```python
from build123d import *

# Parameters (mm, degrees)
SALIENTE_EXTRUIR1_DEPTH = 37
SALIENTE_EXTRUIR2_DEPTH = 2
CROQUIS3_R              = 6.5
SALIENTE_EXTRUIR3_DEPTH = 1
CROQUIS4_R              = 5.5
SALIENTE_EXTRUIR4_DEPTH = 0.5
CROQUIS5_R              = 2.75
SALIENTE_EXTRUIR5_DEPTH = 4
CROQUIS7_W              = 11.5
CROQUIS7_H              = 16.4
SALIENTE_EXTRUIR6_DEPTH = 0.3
REDONDEO1_R             = 0.1
REDONDEO2_R             = 0.5
SALIENTE_EXTRUIR7_START = -8.45
SALIENTE_EXTRUIR7_DEPTH = 2.45
SALIENTE_EXTRUIR8_DEPTH = 0.5
CROQUIS11_W             = 6
CROQUIS11_H             = 2.5
SALIENTE_EXTRUIR9_DEPTH = 5
SALIENTE_EXTRUIR9_DRAFT = -8
CROQUIS12_R             = 1.25
CORTAR_EXTRUIR1_DEPTH   = 5
CHAFL_N1_SIZE           = 0.5


with BuildPart() as part:
    # Croquis1 → Saliente-Extruir1 (new body)
    with BuildSketch(Plane(origin=(0, 0, 0), x_dir=(1, 0, 0), z_dir=(0, 1, 0))):
        with BuildLine():
            Line((1, 0), (39, 0))
            ThreePointArc((39, 0), (39.707106781, 0.292893219), (40, 1))
            Line((40, 1), (40, 18))
            ThreePointArc((40, 18), (39.707106781, 18.707106781), (39, 19))
            Line((39, 19), (1, 19))
            ThreePointArc((1, 19), (0.292893219, 18.707106781), (0, 18))
            Line((0, 18), (0, 1))
            ThreePointArc((0, 1), (0.292893219, 0.292893219), (1, 0))
        make_face()
    extrude(amount=SALIENTE_EXTRUIR1_DEPTH)

    # Croquis2 → Saliente-Extruir2 (add)
    with BuildSketch(Plane(origin=(0, 37, 0), x_dir=(1, 0, 0), z_dir=(0, 1, 0))):
        with BuildLine():
            Line((13.315756806, 18.2), (34.5, 18.2))
            Line((34.5, 18.2), (34.5, 14.5))
            ThreePointArc((34.5, 14.5), (37.18337521, 9.5), (34.5, 4.5))
            Line((34.5, 4.5), (34.5, 0.8))
            Line((34.5, 0.8), (13.315756806, 0.8))
            ThreePointArc((13.315756806, 0.8), (0, 9.5), (13.315756806, 18.2))
        make_face()
    extrude(amount=SALIENTE_EXTRUIR2_DEPTH)

    # Croquis3 → Saliente-Extruir3 (add)
    with BuildSketch(Plane(origin=(0, 39, 0), x_dir=(1, 0, 0), z_dir=(0, 1, 0))):
        with Locations(Location((9.5, 9.5, 0), (0, 0, 270))):
            Circle(CROQUIS3_R)
    extrude(amount=SALIENTE_EXTRUIR3_DEPTH)

    # Croquis4 → Saliente-Extruir4 (add)
    with BuildSketch(Plane(origin=(0, 40, 0), x_dir=(1, 0, 0), z_dir=(0, 1, 0))):
        with Locations(Location((9.5, 9.5, 0), (0, 0, 270))):
            Circle(CROQUIS4_R)
    extrude(amount=SALIENTE_EXTRUIR4_DEPTH)

    # Croquis5 → Saliente-Extruir5 (add)
    with BuildSketch(Plane(origin=(0, 40.5, 0), x_dir=(1, 0, 0), z_dir=(0, 1, 0))):
        with Locations(Location((9.5, 9.5, 0), (0, 0, 270))):
            Circle(CROQUIS5_R)
    extrude(amount=SALIENTE_EXTRUIR5_DEPTH)

    # Croquis7 → Saliente-Extruir6 (add)
    with BuildSketch(Plane(origin=(0, 39, 0), x_dir=(1, 0, 0), z_dir=(0, 1, 0))):
        with BuildLine():
            Line((34.5, 0.8), (22, 0.8))
            Line((22, 0.8), (22, 8))
            ThreePointArc((22, 8), (20.5, 9.5), (22, 11))
            Line((22, 11), (22, 18.2))
            Line((22, 18.2), (34.5, 18.2))
            Line((34.5, 18.2), (34.5, 0.8))
        make_face()
        with Locations((28.25, 9.5)):
            Rectangle(CROQUIS7_W, CROQUIS7_H, mode=Mode.SUBTRACT)
    extrude(amount=SALIENTE_EXTRUIR6_DEPTH)

    # Redondeo1
    redondeo1_edges = [part.edges().sort_by_distance(p)[0] for p in [
        (34, 39.15, -1.3),
        (34, 39.15, -17.7),
        (22.5, 39.15, -17.7),
        (22.5, 39.15, -1.3),
    ]]
    fillet(redondeo1_edges, radius=REDONDEO1_R)

    # Redondeo2
    redondeo2_edges = [part.edges().sort_by_distance(p)[0] for p in [
        (34.5, 38.15, -0.8),
        (34.5, 38.15, -18.2),
    ]]
    fillet(redondeo2_edges, radius=REDONDEO2_R)

    # Croquis8 → Saliente-Extruir7 (add)
    with BuildSketch(Plane(origin=(0, 37, 0), x_dir=(1, 0, 0), z_dir=(0, 1, 0)).offset(SALIENTE_EXTRUIR7_START)):
        with BuildLine():
            Line((40, 1), (40, 18))
            ThreePointArc((40, 18), (39.965925826, 18.258819045), (39.866025404, 18.5))
            Line((39.866025404, 18.5), (45.5, 18.5))
            ThreePointArc((45.5, 18.5), (46.560660172, 18.060660172), (47, 17))
            Line((47, 17), (47, 15))
            ThreePointArc((47, 15), (43.267949192, 14), (47, 13))
            Line((47, 13), (47, 6))
            ThreePointArc((47, 6), (43.267949192, 5), (47, 4))
            Line((47, 4), (47, 2))
            ThreePointArc((47, 2), (46.560660172, 0.939339828), (45.5, 0.5))
            Line((45.5, 0.5), (39.866025404, 0.5))
            ThreePointArc((39.866025404, 0.5), (39.965925826, 0.741180955), (40, 1))
        make_face()
        with BuildLine():
            Line((-7, 17), (-7, 15))
            ThreePointArc((-7, 15), (-3.267949192, 14), (-7, 13))
            Line((-7, 13), (-7, 6))
            ThreePointArc((-7, 6), (-3.267949192, 5), (-7, 4))
            Line((-7, 4), (-7, 2))
            ThreePointArc((-7, 2), (-6.560660172, 0.939339828), (-5.5, 0.5))
            Line((-5.5, 0.5), (0.133974596, 0.5))
            ThreePointArc((0.133974596, 0.5), (0.034074174, 0.741180955), (0, 1))
            Line((0, 1), (0, 18))
            ThreePointArc((0, 18), (0.034074174, 18.258819045), (0.133974596, 18.5))
            Line((0.133974596, 18.5), (-5.5, 18.5))
            ThreePointArc((-5.5, 18.5), (-6.560660172, 18.060660172), (-7, 17))
        make_face()
    extrude(amount=SALIENTE_EXTRUIR7_DEPTH)

    # Croquis10 → Saliente-Extruir8 (add, symmetric)
    with BuildSketch(Plane.XY.offset(-9.5)):
        Polygon((47, 31), (40, 32), (40, 31), align=None)
        Polygon((0, 32), (0, 31), (-7, 31), align=None)
    extrude(amount=SALIENTE_EXTRUIR8_DEPTH, both=True)


with BuildPart() as saliente_extruir9_tool:
    # Croquis11 → Saliente-Extruir9 (with draft: the straight prism first)
    with BuildSketch(Plane(origin=(0, 0, 0), x_dir=(0, 0, -1), z_dir=(1, 0, 0))):
        with Locations((9.5, 4.25)):
            Rectangle(CROQUIS11_W, CROQUIS11_H)
    extrude(amount=-SALIENTE_EXTRUIR9_DEPTH)
    # Saliente-Extruir9: the draft: its side faces are tilted about the plane it starts from
    saliente_extruir9_sides = [saliente_extruir9_tool.faces().sort_by_distance(p)[0] for p in [
        (-2.5, 4.25, -6.5),
        (-2.5, 3, -9.5),
        (-2.5, 4.25, -12.5),
        (-2.5, 5.5, -9.5),
    ]]
    draft(saliente_extruir9_sides, Plane(origin=(0, 0, 0), x_dir=(0, 0, -1), z_dir=(1, 0, 0)), SALIENTE_EXTRUIR9_DRAFT)


with BuildPart() as part_1:
    add(part.part)

    # Saliente-Extruir9: add saliente_extruir9_tool
    add(saliente_extruir9_tool.part)

    # Croquis12 → Cortar-Extruir1 (cut)
    with BuildSketch(Plane(origin=(0, 44.5, 0), x_dir=(1, 0, 0), z_dir=(0, 1, 0))):
        with Locations(Location((9.5, 9.5, 0), (0, 0, 270))):
            Circle(CROQUIS12_R)
    extrude(amount=-CORTAR_EXTRUIR1_DEPTH, mode=Mode.SUBTRACT)

    # Chaflán1
    chafl_n1_edges = [part_1.edges().sort_by_distance(p)[0] for p in [
        (9.5, 44.5, -12.25),
    ]]
    chamfer(chafl_n1_edges, length=CHAFL_N1_SIZE)


solid = part_1.part
```
Check sheet for the modelled part. Datum: model origin and axes. Units: mm. A direction names the side the tool comes from. Give positions to 0.01 mm unless a question says otherwise; leave off trailing zeros. Loops run counter-clockwise (first coordinate to the right, second up) from the corner with the lowest first, then second, coordinate; pieces in that order, holes last. Notation, with made-up numbers: M 87,76 L 92,76 A12 ccw 92,85 Z; hole C 68.5,82.25 d10. An arc over 180 degrees is marked long. Answer in a Markdown table with one row per item.
1) Cross-section at A-A (x = 17.5). Enter the section's corners in (y, z), plus the area to 3 significant figures.
Solutions:
| item | result |
|---|---|
| outline | M 0,-19 L 37,-19 L 37,-18.2 L 39,-18.2 L 39,-0.8 L 37,-0.8 L 37,0 L 0,0 Z |
| area | 738 mm^2 |
2) Mould release check, pull along X, two halves, no side actions. Record for faces 1 (the face through (-3.27, 29.76, -14.07)), 2 (the face through (2, 37, -17)), 3 (the face through (10.345, 42.035, -10.421)), 4 (the face through (40, 14, -9)): released by +X, released by -X, zero draft, split by the parting line, or undercut.
Solutions:
| item | result |
|---|---|
| face 1 | undercut |
| face 2 | zero draft |
| face 3 | undercut |
| face 4 | released by +X |
3) Depth check by flat-ended pin: pin 1 (12 mm diameter, centred on x = -1.5, y = 10, fed in from +Z); pin 2 (10 mm diameter, centred on y = 11.5, z = -12.5, fed in from +X); pin 3 (2 mm diameter, centred on x = 45, z = -15.5, fed in from +Y); pin 4 (0.8 mm diameter, centred on x = 36.5, z = -11, fed in from +Y). Enter the tip coordinate at first touch or a pass-through.
Solutions:
| item | result |
|---|---|
| pin 1 | stops at z = 0 |
| pin 2 | stops at x = 40 |
| pin 3 | stops at y = 31 |
| pin 4 | stops at y = 39 |
4) Cross-section at B-B (y = 16). Enter the section's corners in (x, z).
Solutions:
| item | result |
|---|---|
| outline | M 0,-18 A1 ccw 1,-19 L 39,-19 A1 ccw 40,-18 L 40,-1 A1 ccw 39,0 L 1,0 A1 ccw 0,-1 Z |
5) Thickness scan on line 1 (Y direction, x = 6, z = -3.75); line 2 (Y direction, x = 13.5, z = -12.25); line 3 (X direction, y = 32, z = -4.25). Record the ranges inside material, lowest first.
Solutions:
| item | result |
|---|---|
| line 1 | y = 0 to 39 |
| line 2 | y = 0 to 40.5 |
| line 3 | x = 0 to 40 |
6) Tool access check on faces 5 (the face through (-1.91, 4.23, -6.77)), 6 (the face through (11, 40, -15)), 7 (the face through (24, 38, -0.8)). Record the directions out of +Z, -Z, +X, -X, +Y, -Y that give a thin tool (end or side, any length) a straight path to the whole face; none if there is none.
Solutions:
| item | result |
|---|---|
| face 5 | +Z, -X, -Y |
| face 6 | +Y |
| face 7 | +Z, +X, +Y |
